from build123d import *

# Parameters (mm, degrees)
SKETCH1_R           = 2.5
BOSS_EXTRUDE1_DEPTH = 3
FILLET1_R           = 3


with BuildPart() as part:
    # Sketch1 → Boss-Extrude1 (new body)
    with BuildSketch(Plane(origin=(0, 0, 0), x_dir=(0, 0, -1), z_dir=(1, 0, 0))):
        with BuildLine():
            Line((17.320508076, 0), (40, 0))
            Line((40, 0), (40, 20))
            Line((40, 20), (11.547005384, 20))
            ThreePointArc((11.547005384, 20), (1.547005384, 17.320508076), (-5.773502692, 10))
            Line((-5.773502692, 10), (-28.660254038, -29.641016151))
            Line((-28.660254038, -29.641016151), (-11.339745962, -39.641016151))
            Line((-11.339745962, -39.641016151), (8.660254038, -5))
            ThreePointArc((8.660254038, -5), (12.320508076, -1.339745962), (17.320508076, 0))
        make_face()
        with Locations((-15, -25.980762114)):
            Circle(SKETCH1_R, mode=Mode.SUBTRACT)
        with Locations((-7.5, -12.990381057)):
            Circle(SKETCH1_R, mode=Mode.SUBTRACT)
        with BuildLine():
            Line((19, 12.5), (36, 12.5))
            ThreePointArc((36, 12.5), (38.5, 10), (36, 7.5))
            Line((36, 7.5), (19, 7.5))
            ThreePointArc((19, 7.5), (16.5, 10), (19, 12.5))
        make_face(mode=Mode.SUBTRACT)
    extrude(amount=BOSS_EXTRUDE1_DEPTH)

    # Fillet1
    fillet1_edges = [part.edges().sort_by_distance(p)[0] for p in [
        (1.5, 0, -40),
        (1.5, -39.641016151, 11.339745962),
        (1.5, -29.641016151, 28.660254038),
        (1.5, 20, -40),
    ]]
    fillet(fillet1_edges, radius=FILLET1_R)


solid = part.part
Can you work these out from the model? Positions are in its coordinate system, mm. A direction names the side the tool comes from. Coordinates: 2 decimals unless noted, no trailing zeros. Order: outer loops, then holes, each group sorted by start corner. A loop starts at its lowest first (then second) coordinate and runs counter-clockwise, first axis right, second up. Notation, with made-up numbers: (10, 60.25) - (46, 60.25) arc R30 cw to (46, 84.25) - close; hole circle Ø10 at (-27, 4). An arc over 180 degrees is marked (long way). Answer as a JSON object with one key per item and string values. Group by question number.
Q1. On a 3-axis mill with a long thin cutter (end or side, diameter ignored), from which of +Z, -Z, +X, -X, +Y, -Y can I reach the whole of each face in a straight line? I mean faces 1 (the face through (1.5, 9.9, -16.5)), 2 (the face through (1, 20, -24)), 3 (the face through (1, 0, -27)). Say none if no direction works.
Q2. Imagine slicing it at C-C (z = 15). Please give me the cut outline in (x, y).
Q3. Imagine slicing it at B-B (x = 2.3). Please give me the cut outline in (y, z).
Q4. Imagine slicing it at D-D (y = 1). Please give me the cut outline in (x, z).
Q5. I need wall thicknesses on line 1 (Y direction, x = 0.35, z = -27.5); line 2 (Y direction, x = 2.05, z = 7.5); line 3 (Z direction, x = 0.35, y = -25.5). Which ranges of each line are inside material? Lowest first, please. Write a range as from..to.
Q6. Imagine slicing it at A-A (z = -30). Please give me the cut outline in (x, y).
Q7. We'd pull the mould along X, two halves only. Please class faces 4 (the face through (1, 10, -40)), 5 (the face through (0, -2, -6)), 6 (the face through (3, -2, -6)): +X half, -X half, draft (parallel to the pull), parting line (faces both ways), or undercut.
Q8. Will these pins go through, and if not, where does the flat tip stop? P1, Ø1.5, axis at x = 2, z = -28, coming from the -Y side; P2, Ø1.5, axis at x = 2, y = -21, coming from the +Z side.
Determined:
{
 "1": {"face 1": "+X, -X", "face 2": "+Z, -Z, +X, -X, +Y", "face 3": "-Z, +X, -X, -Y"},
 "2": {"outline": "(0, -37.53) - (3, -37.53) - (3, -28.48) - (0, -28.48) - close; (0, -23.48) - (3, -23.48) - (3, -5.98) - (0, -5.98) - close"},
 "3": {"outline": "(-38.14, 13.94) arc R3 ccw to (-37.04, 9.84) - (-5, -8.66) arc R10 cw to (0, -17.32) - (0, -37) arc R3 ccw to (3, -40) - (17, -40) arc R3 ccw to (20, -37) - (20, -11.55) arc R20 ccw to (10, 5.77) - (-27.04, 27.16) arc R3 ccw to (-31.14, 26.06) - close; hole circle Ø5 at (-25.98, 15); hole circle Ø5 at (-12.99, 7.5); hole (7.5, -36) arc R2.5 ccw to (12.5, -36) - (12.5, -19) arc R2.5 ccw to (7.5, -19) - close"},
 "4": {"outline": "(0, -39.24) - (3, -39.24) - (3, 10.97) - (0, 10.97) - close"},
 "5": {"line 1": "y = 0..7.5, 12.5..20", "line 2": "y = -32.99..-15.49, -10.49..7.01", "line 3": "z = 3.18..12.55, 17.45..26.27"},
 "6": {"outline": "(0, 0) - (3, 0) - (3, 7.5) - (0, 7.5) - close; (0, 12.5) - (3, 12.5) - (3, 20) - (0, 20) - close"},
 "7": {"face 4": "draft", "face 5": "-X half", "face 6": "+X half"},
 "8": {"P1": "stops at y = 0", "P2": "stops at z = 24.1"}
}
